Verification items for the finished model (mm, model axes). Face numbers are marked on the shaded views. A direction names the side the tool comes from. Round coordinates to 2 decimals unless told otherwise and drop trailing zeros. Write each loop counter-clockwise with the first axis right and the second up, starting at its lowest first coordinate (ties: lowest second). Pieces come first, ordered by that corner, then holes. Notation, with made-up numbers: (0, 1) - (30, 1) arc R21 cw to (30, 20) - close; hole circle Ø8 at (11, 84.5). An arc over 180 degrees is marked (long way). Answer as a JSON object with one key per item and string values. Group by question number.
1) Set-up check for the marked faces 4 and 5: record each of +Z, -Z, +X, -X, +Y, -Y from which the full face is reachable in a straight line by a thin tool's end or side.
2) Section check D-D (z = -13). Enter the section's corners in (x, y), then the cut area to 3 significant figures.
3) Section check C-C (x = 13). Enter the section's corners in (y, z), then the cut area to 3 significant figures.
4) Section check A-A (y = 0). Enter the section's corners in (x, z), then the cut area to 3 significant figures.
5) Section check B-B (z = -29.5). Enter the section's corners in (x, y).
6) Go/stop test with a flat-tipped pin: pin 1 Ø1.5 at (x, y) = (3, -6) entering from +Z. Record where the tip stops, or that it passes through.
7) Thickness scan on line 1 (Z direction, x = 18.9, y = 0); line 2 (X direction, y = -2.5, z = -21.5); line 3 (Y direction, x = -18.4, z = 0). Record the ranges inside material, lowest first.
8) Mould release check, pull along X, two halves, no side actions. Record for the marked faces 1, 2 and 3: +X half, -X half, draft (parallel to the pull), parting line (faces both ways), or undercut.
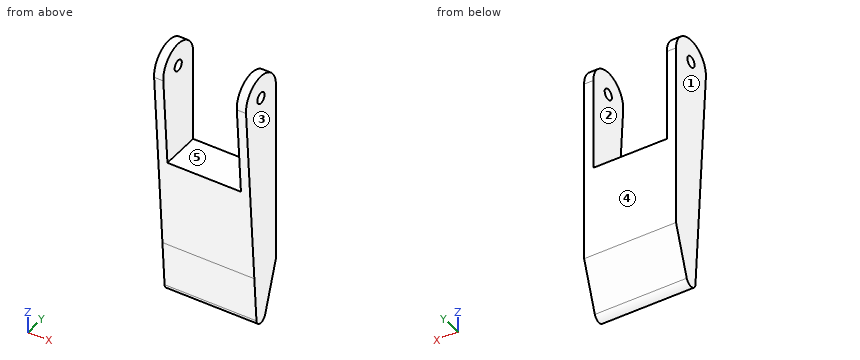
```python
from build123d import *

# Parameters (mm, degrees)
SKETCH1_R              = 2.4
ARM_DEPTH              = 20
ELBOW_MOUNT_DEPTH      = 106.399240984
ELBOW_MOUNT_DEPTH_BACK = 106.399240984
SKETCH2_W              = 32
SKETCH2_H              = 50


with BuildPart() as part:
    # Sketch1 → arm (new, symmetric)
    with BuildSketch(Plane(origin=(0, 0, 0), x_dir=(0, 0, -1), z_dir=(1, 0, 0))):
        with BuildLine():
            Line((0, 10), (80, 10))
            Line((80, 10), (100.969511188, 2.839022377))
            ThreePointArc((100.969511188, 2.839022377), (102.974875799, -0.387445454), (100.21, -2.992640974))
            Line((100.21, -2.992640974), (80, -4.410819779))
            Line((80, -4.410819779), (0.7, -9.975469914))
            ThreePointArc((0.7, -9.975469914), (-9.993865597, -0.350214836), (0, 10))
        make_face()
        Circle(SKETCH1_R, mode=Mode.SUBTRACT)
    extrude(amount=ARM_DEPTH, both=True)

    # Sketch2 → elbow mount (cut, two sides: drawn at the far end of the back side and taken through both)
    with BuildSketch(Plane(origin=(0, 0, 0), x_dir=(1, 0, 0), z_dir=(0, 1, 0)).offset(-ELBOW_MOUNT_DEPTH_BACK)):
        with Locations((0, 15)):
            Rectangle(SKETCH2_W, SKETCH2_H)
    extrude(amount=ELBOW_MOUNT_DEPTH + ELBOW_MOUNT_DEPTH_BACK, mode=Mode.SUBTRACT)


solid = part.part
```
Returned:
{
 "1": {"face 4": "+Z, -Z, +X, -X, +Y", "face 5": "+Z, +Y, -Y"},
 "2": {"outline": "(-20, -9.11) - (-16, -9.11) - (-16, 10) - (-20, 10) - close; (16, -9.11) - (20, -9.11) - (20, 10) - (16, 10) - close", "area": "153 mm2"},
 "3": {"outline": "(-7.22, -40) - (-2.99, -100.21) arc R3 ccw to (2.84, -100.97) - (10, -80) - (10, -40) - close", "area": "853 mm2"},
 "4": {"outline": "(-20, -103) - (20, -103) - (20, -2.4) - (16, -2.4) - (16, -40) - (-16, -40) - (-16, -2.4) - (-20, -2.4) - close; (-20, 2.4) - (-16, 2.4) - (-16, 10) - (-20, 10) - close; (16, 2.4) - (20, 2.4) - (20, 10) - (16, 10) - close", "area": "2,880 mm2"},
 "5": {"outline": "(-20, -7.95) - (-16, -7.95) - (-16, 10) - (-20, 10) - close; (16, -7.95) - (20, -7.95) - (20, 10) - (16, 10) - close"},
 "6": {"pin 1": "z = -40"},
 "7": {"line 1": "-103 to -2.4, 2.4 to 10", "line 2": "-20 to -16, 16 to 20", "line 3": "-10 to -2.4, 2.4 to 10"},
 "8": {"face 1": "-X half", "face 2": "undercut", "face 3": "+X half"}
}
